```python
from build123d import *

# Parameters (mm, degrees)
SKETCH_1_W          = 38
SKETCH_1_H          = 10
EXTRUDE_1_DEPTH     = 1
FILLET_1_R          = 1
SKETCH_2_R          = 1.5
CUT_EXTRUDE_1_DEPTH = 20.672315573
SKETCH_3_W          = 2.5
SKETCH_3_H          = 0.5
CUT_EXTRUDE_2_DEPTH = 0.5


with BuildPart() as part:
    # Эскиз1 → Бобышка-Вытянуть1 (new body)
    with BuildSketch(Plane(origin=(0, 0, 0), x_dir=(1, 0, 0), z_dir=(0, 1, 0))):
        Rectangle(SKETCH_1_W, SKETCH_1_H)
    extrude(amount=EXTRUDE_1_DEPTH)

    # Скругление1
    fillet_1_edges = [part.edges().sort_by_distance(p)[0] for p in [
        (19, 0.5, 5),
        (-19, 0.5, 5),
        (-19, 0.5, -5),
        (19, 0.5, -5),
    ]]
    fillet(fillet_1_edges, radius=FILLET_1_R)

    # Эскиз2 → Вырез-Вытянуть1 (cut, through all)
    with BuildSketch(Plane(origin=(0, 1, 0), x_dir=(1, 0, 0), z_dir=(0, 1, 0))):
        with Locations(Location((-13.5, 0, 0), (0, 0, 270))):
            Circle(SKETCH_2_R)
        with Locations(Location((-4.5, 0, 0), (0, 0, 270))):
            Circle(SKETCH_2_R)
        with Locations(Location((4.5, 0, 0), (0, 0, 270))):
            Circle(SKETCH_2_R)
        with Locations(Location((13.5, 0, 0), (0, 0, 270))):
            Circle(SKETCH_2_R)
    extrude(amount=-CUT_EXTRUDE_1_DEPTH, mode=Mode.SUBTRACT)

    # Эскиз3 → Вырез-Вытянуть2 (cut)
    with BuildSketch(Plane(origin=(0, 1, 0), x_dir=(1, 0, 0), z_dir=(0, 1, 0))):
        Polygon((0, 2.5), (0, 1.5), (-0.5, 1.5), (-0.5, 2.5), (-1.5, 2.5), (-1.5, 3), (-0.5, 3), (-0.5, 4), (0, 4), (0, 3), (1, 3), (1, 2.5), align=None)
        with Locations((-8.75, 2.75)):
            Rectangle(SKETCH_3_W, SKETCH_3_H)
    extrude(amount=-CUT_EXTRUDE_2_DEPTH, mode=Mode.SUBTRACT)


solid = part.part
```
Check sheet for the modelled part. Datum: model origin and axes. Units: mm. Give positions to 0.01 mm unless a question says otherwise; leave off trailing zeros. Order: outer loops, then holes, each group sorted by start corner. A loop starts at its lowest first (then second) coordinate and runs counter-clockwise, first axis right, second up. Notation, with made-up numbers: M 60.25,1 L 79.25,1 A30 ccw 79.25,29 Z; hole C -15.75,-10 d6. An arc over 180 degrees is marked long. Answer in a Markdown table with one row per item.
1) Cross-section at A-A, the plane y = 0.8. Enter the section's corners in (x, z), plus the area to 3 significant figures.
Filled sheet:
| item | result |
|---|---|
| outline | M -19,-4 A1 ccw -18,-5 L 18,-5 A1 ccw 19,-4 L 19,4 A1 ccw 18,5 L -18,5 A1 ccw -19,4 Z; hole C -13.5,0 d3; hole M -10,-3 L -7.5,-3 L -7.5,-2.5 L -10,-2.5 Z; hole C -4.5,0 d3; hole M -1.5,-3 L -0.5,-3 L -0.5,-4 L 0,-4 L 0,-3 L 1,-3 L 1,-2.5 L 0,-2.5 L 0,-1.5 L -0.5,-1.5 L -0.5,-2.5 L -1.5,-2.5 Z; hole C 4.5,0 d3; hole C 13.5,0 d3 |
| area | 347 mm2 |
2) Gauge pin test, flat end, axial feed: P1, Ø2.5, axis at x = 13.5, z = 0, coming from the +Y side. Record the tip position at first contact, or that the pin passes through.
Filled sheet:
| item | result |
|---|---|
| P1 | passes through |
3) Cross-section at B-B, the plane z = 0. Enter the section's corners in (x, y).
Filled sheet:
| item | result |
|---|---|
| outline | M -19,0 L -15,0 L -15,1 L -19,1 Z; M -12,0 L -6,0 L -6,1 L -12,1 Z; M -3,0 L 3,0 L 3,1 L -3,1 Z; M 6,0 L 12,0 L 12,1 L 6,1 Z; M 15,0 L 19,0 L 19,1 L 15,1 Z |
4) Cross-section at D-D, the plane x = 13.5. Enter the section's corners in (y, z).
Filled sheet:
| item | result |
|---|---|
| outline | M 0,-5 L 1,-5 L 1,-1.5 L 0,-1.5 Z; M 0,1.5 L 1,1.5 L 1,5 L 0,5 Z |
5) Thickness scan on L1, parallel to X at y = 0.85, z = 0; L2, parallel to X at y = 0.25, z = 1; L3, parallel to X at y = 0.7, z = -3.75. Record the ranges inside material, lowest first. Write a range as [from, to].
Filled sheet:
| item | result |
|---|---|
| L1 | x = [-19, -15], [-12, -6], [-3, 3], [6, 12], [15, 19] |
| L2 | x = [-19, -14.62], [-12.38, -5.62], [-3.38, 3.38], [5.62, 12.38], [14.62, 19] |
| L3 | x = [-19, -0.5], [0, 19] |
6) Cross-section at C-C, the plane x = -9. Enter the section's corners in (y, z), plus the area to 3 significant figures.
Filled sheet:
| item | result |
|---|---|
| outline | M 0,-5 L 1,-5 L 1,-3 L 0.5,-3 L 0.5,-2.5 L 1,-2.5 L 1,5 L 0,5 Z |
| area | 9.75 mm2 |
